Work out the finished part from the listing and answer in its coordinate system (mm). Face numbers are marked on the shaded views. Give positions to 0.01 mm unless a question says otherwise; leave off trailing zeros. Order: outer loops, then holes, each group sorted by start corner. A loop starts at its lowest first (then second) coordinate and runs counter-clockwise, first axis right, second up.
```python
from build123d import *

# Parameters (mm, degrees)
F0_R     = 11
F1_DEPTH = 7
F2_R     = 15


with BuildPart() as f1:
    # F0 (on Top) → F1 (new body)
    with BuildSketch(Plane.XY):
        with BuildLine():
            ThreePointArc((-14.7729482501, -2.6), (-14.9420444362, -1.3173109227), (-14.9999794627, -0.0248217267))
            ThreePointArc((-14.9999794627, -0.0248217267), (-29.1846096908, -16.8497422612), (-7.5214859773, -12.9779524076))
            ThreePointArc((-7.5214859773, -12.9779524076), (-8.6118469419, -12.2815346048), (-9.6381401749, -11.4937484734))
            Line((-9.6381401749, -11.4937484734), (-14.2028166221, -19.4))
            Line((-14.2028166221, -19.4), (-23.9023011445, -19.4))
            Line((-23.9023011445, -19.4), (-28.7520434056, -11))
            Line((-28.7520434056, -11), (-23.9023011445, -2.6))
            Line((-23.9023011445, -2.6), (-14.7729482501, -2.6))
        make_face()
        with BuildLine():
            ThreePointArc((14.9999794627, -0.0248217267), (14.9999948657, -0.0124108676), (15, 0))
            ThreePointArc((15, 0), (12.9841711765, 7.5107455595), (7.4784934854, 13.0027741343))
            ThreePointArc((7.4784934854, 13.0027741343), (6.3301974943, 13.5988455276), (5.1348080752, 14.0937484734))
            Line((5.1348080752, 14.0937484734), (4.8497422612, 13.6))
            Line((4.8497422612, 13.6), (-4.8497422612, 13.6))
            Line((-4.8497422612, 13.6), (-5.1348080752, 14.0937484734))
            ThreePointArc((-5.1348080752, 14.0937484734), (-6.3301974943, 13.5988455276), (-7.4784934854, 13.0027741343))
            ThreePointArc((-7.4784934854, 13.0027741343), (-12.9903810568, 7.5), (-14.9999794627, -0.0248217267))
            ThreePointArc((-14.9999794627, -0.0248217267), (-14.9420444362, -1.3173109227), (-14.7729482501, -2.6))
            Line((-14.7729482501, -2.6), (-14.2028166221, -2.6))
            Line((-14.2028166221, -2.6), (-9.3530743609, -11))
            Line((-9.3530743609, -11), (-9.6381401749, -11.4937484734))
            ThreePointArc((-9.6381401749, -11.4937484734), (-8.6118469419, -12.2815346048), (-7.5214859773, -12.9779524076))
            ThreePointArc((-7.5214859773, -12.9779524076), (0, -15), (7.5214859773, -12.9779524076))
            ThreePointArc((7.5214859773, -12.9779524076), (8.6118469419, -12.2815346048), (9.6381401749, -11.4937484734))
            Line((9.6381401749, -11.4937484734), (9.3530743609, -11))
            Line((9.3530743609, -11), (14.2028166221, -2.6))
            Line((14.2028166221, -2.6), (14.7729482501, -2.6))
            ThreePointArc((14.7729482501, -2.6), (14.9420444362, -1.3173109227), (14.9999794627, -0.0248217267))
        make_face()
        Circle(F0_R, mode=Mode.SUBTRACT)
        with BuildLine():
            ThreePointArc((7.5214859773, -12.9779524076), (29.1846096908, -16.8497422612), (14.9999794627, -0.0248217267))
            ThreePointArc((14.9999794627, -0.0248217267), (14.9420444362, -1.3173109227), (14.7729482501, -2.6))
            Line((14.7729482501, -2.6), (23.9023011445, -2.6))
            Line((23.9023011445, -2.6), (28.7520434056, -11))
            Line((28.7520434056, -11), (23.9023011445, -19.4))
            Line((23.9023011445, -19.4), (14.2028166221, -19.4))
            Line((14.2028166221, -19.4), (9.6381401749, -11.4937484734))
            ThreePointArc((9.6381401749, -11.4937484734), (8.6118469419, -12.2815346048), (7.5214859773, -12.9779524076))
        make_face()
        with BuildLine():
            ThreePointArc((5.1348080752, 14.0937484734), (6.3301974943, 13.5988455276), (7.4784934854, 13.0027741343))
            ThreePointArc((7.4784934854, 13.0027741343), (0, 33.6994845224), (-7.4784934854, 13.0027741343))
            ThreePointArc((-7.4784934854, 13.0027741343), (-6.3301974943, 13.5988455276), (-5.1348080752, 14.0937484734))
            Line((-5.1348080752, 14.0937484734), (-9.6994845224, 22))
            Line((-9.6994845224, 22), (-4.8497422612, 30.4))
            Line((-4.8497422612, 30.4), (4.8497422612, 30.4))
            Line((4.8497422612, 30.4), (9.6994845224, 22))
            Line((9.6994845224, 22), (5.1348080752, 14.0937484734))
        make_face()
    extrude(amount=F1_DEPTH)

    # F2
    f2_edges = [f1.edges().sort_by_distance(p)[0] for p in [
        (7.521486, -12.977952, 3.5),
        (-14.999979, -0.024822, 3.5),
        (7.478493, 13.002774, 3.5),
        (-7.521486, -12.977952, 3.5),
        (14.999979, -0.024822, 3.5),
        (-7.478493, 13.002774, 3.5),
    ]]
    fillet(f2_edges, radius=F2_R)


solid = f1.part
```
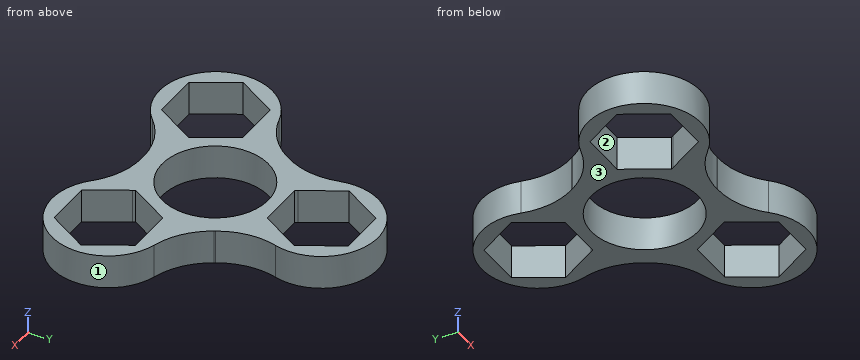
1. The mould has two halves that part along Y. Classify the marked faces 1, 2 and 3: pulls with the +Y half, pulls with the -Y half, needs draft (parallel to the pull), parting line crosses it, or undercut.
Findings below:
face 1: parting line crosses it
face 2: undercut
face 3: needs draft
2. The part is cut by section A-A (y = 29.5). Write down the section's boundary in (x, z), then the cut area to 3 significant figures.
Findings below:
outline: (-8.98, 0) - (-5.37, 0) - (-5.37, 7) - (-8.98, 7) - close; (5.37, 0) - (8.98, 0) - (8.98, 7) - (5.37, 7) - close
area: 50.5 mm2
3. Straight lines are drawn through the part: probe 1 along X at (y, z) = (-4.5, 2.5); probe 2 along Y at (x, z) = (6, 4.5); probe 3 along Y at (x, z) = (3.5, 6.5). For each, find the intervals that lie inside material, in ascending order.
Findings below:
probe 1: x = -28.78 to -25, -13.11 to -10.04, 10.04 to 13.11, 25 to 28.78
probe 2: y = -16.13 to -9.22, 9.22 to 15.59, 28.41 to 32.04
probe 3: y = -15.35 to -10.43, 10.43 to 13.6, 30.4 to 33.16
4. Given P1, Ø17.5, axis at x = 0, y = 0, coming from the -Z side; P2, Ø1.5, axis at y = 13, z = 4.5, coming from the +X side; P3, Ø3.5, axis at x = -2, z = 4.5, coming from the -Y side; P4, Ø3, axis at x = -5, z = 3, coming from the -Y side, each flat-ended and moving along its own axis, determine where each tip first touches the part or whether it passes through.
Findings below:
P1: passes through
P2: stops at x = 11.14
P3: stops at y = -15.4
P4: stops at y = -16.34
5. The part is cut by section B-B (x = -6.5). State how many separate pieces and enclosed holes the cut face has, then the cut area to 3 significant figures.
Findings below:
separate pieces: 3
enclosed holes: 0
area: 135 mm2
